Autodesk Inventor part; units mm, degrees
ref_plane "YZ Plane" through (0, 0, 0) normal (1, 0, 0) x (0, 1, 0)
ref_plane "XZ Plane" through (0, 0, 0) normal (0, 1, 0) x (-1, 0, 0)
ref_plane "XY Plane" through (0, 0, 0) normal (0, 0, 1) x (1, 0, 0)
sketch "Sketch1" plane through (0, 0, 0) normal (0, 0, 1) x (1, 0, 0)
  line L0 (21.5871, 13.6345) -> (17.0871, 18.1345)
  line L1 (17.0871, 18.1345) -> (-16.7129, 18.1345)
  line L2 (-16.7129, 18.1345) -> (-21.2129, 13.6345)
  line L3 (-21.0966, 13.6345) -> (-21.0966, -20.1655)
  line L4 (21.4709, -20.1655) -> (21.4709, 13.6345)
  line L5 (21.4709, -20.1655) -> (17.0871, -24.4078)
  line L6 (-16.7129, -24.4078) -> (17.0871, -24.4078)
  line L7 (-16.7129, -24.4078) -> (-21.0966, -20.1655)
  line L8 (-24.7129, -28.1655) -> (-24.7129, 13.6345) construction
  line L9 (25.0871, -28.1655) -> (-24.7129, -28.1655) construction
  line L10 (25.0871, -28.1655) -> (25.0871, 13.6345) construction
  line L11 (17.0871, 21.6345) -> (-16.7129, 21.6345) construction
  line L12 (-21.0552, -20.0655) -> (-16.6129, -24.5078)
  line L13 (-16.6129, -24.5078) -> (-16.6129, -28.1655)
  line L14 (-16.6129, -28.1655) -> (17.0871, -28.1655)
  line L15 (25.0871, -20.0655) -> (21.4295, -20.0655)
  line L16 (25.0871, 13.5345) -> (25.0871, -20.0655)
  line L17 (21.4295, 13.5345) -> (25.0871, 13.5345)
  line L18 (21.4295, 13.5345) -> (16.9871, 17.9768)
  line L19 (16.9871, 17.9768) -> (16.9871, 21.6345)
  line L20 (16.9871, 21.6345) -> (-16.6129, 21.6345)
  line L21 (-16.6129, 21.6345) -> (-16.6129, 17.9768)
  line L22 (-16.6129, 17.9768) -> (-21.0552, 13.5345)
  line L23 (-24.7129, 13.5345) -> (-21.0552, 13.5345)
  line L24 (-24.7129, -20.0655) -> (-24.7129, 13.5345)
  line L25 (-21.0552, -20.0655) -> (-24.7129, -20.0655)
  line L26 (-12.3129, -23.2655) -> (12.6871, -23.2655)
  line L27 (12.6871, -23.2655) -> (12.6871, 16.7345)
  line L28 (-12.3129, 16.7345) -> (12.6871, 16.7345)
  line L29 (-12.3129, -23.2655) -> (-12.3129, 16.7345)
  line L30 (14.6871, -25.2655) -> (-14.3129, -25.2655) construction
  line L31 (-14.3129, -25.2655) -> (-14.3129, 18.7345) construction
  line L32 (-14.3129, 18.7345) -> (14.6871, 18.7345) construction
  line L33 (14.6871, 18.7345) -> (14.6871, -25.2655) construction
  line L34 (-17.3129, 21.7345) -> (17.6871, 21.7345) construction
  line L35 (17.6871, 21.7345) -> (17.6871, -28.2655) construction
  line L36 (17.6871, -28.2655) -> (-17.3129, -28.2655) construction
  line L37 (-17.3129, -28.2655) -> (-17.3129, 21.7345) construction
  line L38 (-14.3129, -23.2655) -> (-14.3129, -25.2655)
  line L39 (-14.3129, -25.2655) -> (14.6871, -25.2655)
  line L40 (14.6871, -25.2655) -> (14.6871, -20.0655)
  line L41 (14.6871, -20.0655) -> (17.6871, -20.0655)
  line L42 (17.6871, -20.0655) -> (17.6871, 13.5345)
  line L43 (17.6871, 13.5345) -> (14.6871, 13.5345)
  line L44 (14.6871, 13.5345) -> (14.6871, 18.7345)
  line L45 (14.6871, 18.7345) -> (-14.3129, 18.7345)
  line L46 (-14.3129, 18.7345) -> (-14.3129, 13.5345)
  line L47 (-14.3129, 13.5345) -> (-17.3129, 13.5345)
  line L48 (-17.3129, 13.5345) -> (-17.3129, -20.0655)
  line L49 (-17.3129, -20.0655) -> (-14.3129, -20.0655)
  line L50 (-14.3129, -20.0655) -> (-14.3129, -23.2655)
  line L51 (-16.6129, -28.1655) -> (17.0871, -28.1655)
  line L52 (16.9871, -28.1655) -> (16.9871, -24.3509)
  line L53 (16.9871, -24.3509) -> (21.2726, -20.0655)
  line L54 (21.2726, -20.0655) -> (21.4295, -20.0655)
  point P0 (14.2, -44.8454)
  point P1 (16.9871, 19.8057)
  dimension "d74" = 2
  dimension "d75" = 5
  dimension "d76" = 135
extrude "Extrusion1" add sketch "Sketch1" along normal blind 5 contours L19 L18 L17 L4 L15 L54 L53 L52 L6 L40 L41 L42 L43 L44 L1 | L1 L44 L45 L46 L21 L20 L19 | L46 L47 L48 L49 L50 L38 L6 L12 L25 L3 L23 L22 L21 L1 | L17 L16 L15 L4 | L3 L25 L24 L23 | L6 L52 L14 L13 L12 L38 L39 L40
sketch "Sketch5" plane through (0, 0, 0) normal (0, 0, -1) x (-1, 0, 0)
  line L0 (12.3129, -23.2655) -> (-12.6871, -23.2655) construction
  line L1 (-12.6871, -23.2655) -> (-12.6871, 16.7345) construction
  line L2 (12.3129, 16.7345) -> (-12.6871, 16.7345) construction
  line L3 (12.3129, -23.2655) -> (12.3129, 16.7345) construction
  line L4 (-14.6871, -25.2655) -> (14.3129, -25.2655) construction
  arc A0 (14.3129, -25.2655) -> (-0.1871, -22.4693) centre (0.3594, -58.629) ccw
  arc A1 (12.3827, -25.2655) -> (-0.1871, -23.1694) centre (0.3594, -58.629) ccw
  line L5 (-0.1871, -22.4693) -> (-0.1871, -23.1694)
  line L6 (14.3129, -20.0655) -> (14.3129, -25.2655)
  line L7 (14.3129, -25.2655) -> (12.3827, -25.2655)
  point P0 (0, 0)
  dimension "d79" = 0.7
extrude "Extrusion4" add sketch "Sketch5" against normal up to surface (5 mm away)
mirror "Mirror1" about plane through (0.1871, -23.1694, 0) normal (1, 0, 0) of "Extrusion4"
ref_plane "Work Plane1" through (0.1871, -20.0655, 0) normal (-1, 0, 0) x (0, 0, 1)
ref_plane "Work Plane2" through (-16.6129, -3.2655, 0) normal (0, -1, 0) x (1, 0, 0)
mirror "Mirror2" about plane through (-16.6129, -3.2655, 0) normal (0, -1, 0) of "Extrusion4", "Mirror1"
sketch "Sketch6" plane through (0, 0, 0) normal (0, 0, -1) x (-1, 0, 0)
  spline S0 degree 3 poles (1.425, -3.2655) (1.425, -3.4679) (1.3845, -3.6839) (1.22, -4.081) (1.0959, -4.2623) (0.8097, -4.5486) (0.6284, -4.6726) (0.2312, -4.8371) (0.0153, -4.8776) (-0.3896, -4.8776) (-0.6055, -4.8371) (-1.0027, -4.6726) (-1.1839, -4.5486) (-1.4702, -4.2623) (-1.5943, -4.081) (-1.7588, -3.6839) (-1.7992, -3.4679) (-1.7992, -3.0631) (-1.7588, -2.8471) (-1.5943, -2.45) (-1.4702, -2.2687) (-1.1839, -1.9824) (-1.0027, -1.8584) (-0.6055, -1.6939) (-0.3896, -1.6534) (0.0153, -1.6534) (0.2312, -1.6939) (0.6284, -1.8584) (0.8097, -1.9824) (1.0959, -2.2687) (1.22, -2.45) (1.3845, -2.8471) (1.425, -3.0631) (1.425, -3.2655) knots 0 0 0 0 0.060733 0.060733 0.121465 0.121465 0.182198 0.182198 0.24293 0.24293 0.303663 0.303663 0.364395 0.364395 0.425128 0.425128 0.48586 0.48586 0.546593 0.546593 0.607326 0.607326 0.668058 0.668058 0.728791 0.728791 0.789523 0.789523 0.850256 0.850256 0.910988 0.910988 0.971721 0.971721 0.971721 0.971721
  line L0 (17.3129, 13.5345) -> (17.3129, -20.0655)
  arc A0 (13.2973, -3.2655) -> (17.3129, -20.0655) centre (48.9305, -3.6282) ccw
  line L1 (17.3129, -20.0655) -> (14.3129, -20.0655)
  arc A1 (11.9598, -3.2655) -> (15.8129, -20.0655) centre (48.9305, -3.6282) ccw
  line L2 (11.9598, -3.2655) -> (13.2973, -3.2655)
  line L3 (15.8129, -20.0655) -> (17.3129, -20.0655)
  point P0 (0, 0)
  point P1 (1.425, -3.2655)
extrude "Extrusion5" add sketch "Sketch6" against normal up to surface (5 mm away) contours A0 L1 A1 L2
mirror "Mirror3" about plane through (-11.9598, -3.2655, 0) normal (0, 1, 0) of "Extrusion5"
mirror "Mirror4" about plane through (0.1871, -20.0655, 0) normal (-1, 0, 0) of "Extrusion5", "Mirror3"
properties part number "20_Cube_Insert_Lens_Cylindrical"
The listing builds one solid part. Answer for the finished solid, in the listing's coordinates (mm). A direction names the side the tool comes from. Give positions to 0.01 mm unless a question says otherwise; leave off trailing zeros. Loops run counter-clockwise (first coordinate to the right, second up) from the corner with the lowest first, then second, coordinate; pieces in that order, holes last. Notation, with made-up numbers: (24.5, 83) - (80.5, 83) arc R13 cw to (80.5, 89) - close; hole circle Ø3 at (41.25, 55). An arc over 180 degrees is marked (long way). Use one line per item in the form item = value.
1. Section B-B on y = 5 is taken. Give the vertices of the cut face in (x, z).
Calculated:
outline = (-24.71, 0) - (-17.31, 0) - (-17.31, 5) - (-24.71, 5) - close; (-14.18, 0) - (-12.81, 0) - (-12.81, 5) - (-14.18, 5) - close; (13.19, 0) - (14.56, 0) - (14.56, 5) - (13.19, 5) - close; (17.69, 0) - (25.09, 0) - (25.09, 5) - (17.69, 5) - close
2. The mould has two halves that part along Y. Classify faces 1 (the face through (16.987, -26, 2)), 2 (the face through (0, -28.166, 2)), 3 (the face through (-12.867, -11.774, 2.465)): pulls with the +Y half, pulls with the -Y half, needs draft (parallel to the pull), parting line crosses it, or undercut.
Calculated:
face_1 = needs draft
face_2 = pulls with the -Y half
face_3 = undercut
3. Section C-C on z = 1.35 is taken. Count the separate pieces of the cut face and the enclosed holes in it, then the cut area to 3 significant figures.
Calculated:
separate_pieces = 1
enclosed_holes = 5
area = 911 mm^2
4. Given pin 1 Ø8 at (x, y) = (6, 13) entering from +Z; pin 2 Ø2.5 at (y, z) = (-21.5, 3) entering from +X; pin 3 Ø1.8 at (x, z) = (-22, 3) entering from +Y; pin 4 Ø1.1 at (y, z) = (19, 2.5) entering from -X, each flat-ended and moving along its own axis, determine where each tip first touches the part or whether it passes through.
Calculated:
pin_1 = 5
pin_2 = 21.09
pin_3 = 13.53
pin_4 = -16.61
5. Which of the six approach directions +Z, -Z, +X, -X, +Y, -Y give full straight-line access (tool end or side, diameter ignored) to faces 4 (the face through (-23, 13.534, 2)), 5 (the face through (-17.313, -3, 2)), 6 (the face through (16.987, 20, 2)), 7 (the face through (13, -3, 5)), 8 (the face through (-16.613, -26, 2))?
Calculated:
face_4 = +Z, -Z, -X, +Y
face_5 = +Z, -Z
face_6 = +Z, -Z, +X, +Y
face_7 = +Z, +X, -X, +Y, -Y
face_8 = +Z, -Z, -X, -Y
6. Section A-A on x = -5.5 is taken. Give the vertices of the cut face in (y, z).
Calculated:
outline = (-28.17, 0) - (-25.27, 0) - (-25.27, 5) - (-28.17, 5) - close; (-23.54, 0) - (-22.83, 0) - (-22.83, 5) - (-23.54, 5) - close; (16.3, 0) - (17.01, 0) - (17.01, 5) - (16.3, 5) - close; (18.73, 0) - (21.63, 0) - (21.63, 5) - (18.73, 5) - close
7. Find the intervals of material crossed by line 1 along Y through (x, z) = (0.5, 3.4); line 2 along Y through (x, z) = (3, 3.5); line 3 along X through (y, z) = (7, 4.55), in increasing order. Write a range as [from, to].
Calculated:
line_1 = [-28.17, -25.27], [-23.17, -22.47], [15.93, 16.63], [18.73, 21.63]
line_2 = [-28.17, -25.27], [-23.24, -22.54], [16.01, 16.71], [18.73, 21.63]
line_3 = [-24.71, -17.31], [-14.7, -13.31], [13.68, 15.07], [17.69, 25.09]
